Check sheet for the drawn part. Datum: minimum x, y, z corner. Units: mm. Give positions to 0.01 mm unless a question says otherwise; leave off trailing zeros. Order: outer loops, then holes, each group sorted by start corner. A loop starts at its lowest first (then second) coordinate and runs counter-clockwise, first axis right, second up. Notation, with made-up numbers: (78.5, 71.25) - (120.5, 71.25) arc R23 cw to (120.5, 102.25) - close; hole circle Ø9 at (77.25, 55). An arc over 180 degrees is marked (long way). Answer as a JSON object with one key per item and string values. Group by question number.
(1) Thickness scan on line 1 (X direction, y = 19.5, z = 2.75); line 2 (Y direction, x = 21, z = 0.7); line 3 (Y direction, x = 30, z = 2.25). Record the ranges inside material, lowest first.
(2) Section check B-B (x = 14). Record the boundary of the cut face in (y, z).
(3) Section check A-A (z = 0.7). Count the separate pieces of the cut face and the enclosed holes in it, then the cut area to 3 significant figures.
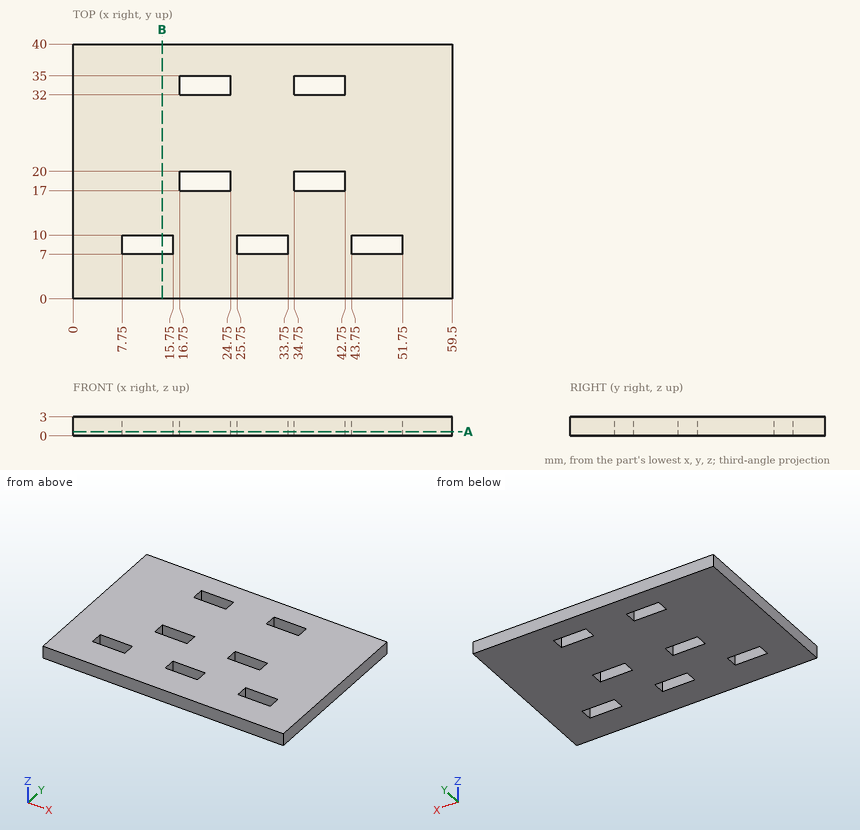
Solutions:
{
 "1": {"line 1": "x = 0 to 16.75, 24.75 to 34.75, 42.75 to 59.5", "line 2": "y = 0 to 17, 20 to 32, 35 to 40", "line 3": "y = 0 to 7, 10 to 40"},
 "2": {"outline": "(0, 0) - (7, 0) - (7, 3) - (0, 3) - close; (10, 0) - (40, 0) - (40, 3) - (10, 3) - close"},
 "3": {"separate pieces": "1", "enclosed holes": "7", "area": "2,210 mm2"}
}
